Geometry: final body of the model. Coordinates: model frame, mm. Face numbers are marked on the shaded views. A direction names the side the tool comes from. Round coordinates to 2 decimals unless told otherwise and drop trailing zeros. Loops run counter-clockwise (first coordinate to the right, second up) from the corner with the lowest first, then second, coordinate; pieces in that order, holes last. Notation, with made-up numbers: (-32.75, 2) - (25.25, 2) arc R14 ccw to (25.25, 11) - close; hole circle Ø8 at (-13.5, -9). An arc over 180 degrees is marked (long way). Answer as CSV lines item,"result".
from build123d import *

# Parameters (mm, degrees)
SKETCH1_R           = 8
BOSS_EXTRUDE1_DEPTH = 3.4
SKETCH2_R           = 8
SKETCH2_R_2         = 7.6
SKETCH2_R_3         = 3.25
BOSS_EXTRUDE2_DEPTH = 1.5


with BuildPart() as part:
    # Sketch1 → Boss-Extrude1 (new body)
    with BuildSketch(Plane(origin=(0, 0, 0), x_dir=(1, 0, 0), z_dir=(0, 1, 0))):
        with Locations(Location((0, 0, 0), (0, 0, 270))):
            Circle(SKETCH1_R)
    extrude(amount=BOSS_EXTRUDE1_DEPTH)

    # Sketch2 → Boss-Extrude2 (add)
    # profile 1 of 2: a face of its own
    with BuildSketch(Plane(origin=(0, 3.4, 0), x_dir=(1, 0, 0), z_dir=(0, 1, 0))):
        with Locations(Location((0, 0, 0), (0, 0, 270))):
            Circle(SKETCH2_R)
        with Locations(Location((0, 0, 0), (0, 0, 270))):
            Circle(SKETCH2_R_2, mode=Mode.SUBTRACT)
    # profile 2 of 2: a face of its own
    with BuildSketch(Plane(origin=(0, 3.4, 0), x_dir=(1, 0, 0), z_dir=(0, 1, 0))):
        with Locations(Location((0, 0, 0), (0, 0, 270))):
            Circle(SKETCH2_R_3)
    extrude(amount=BOSS_EXTRUDE2_DEPTH)


solid = part.part
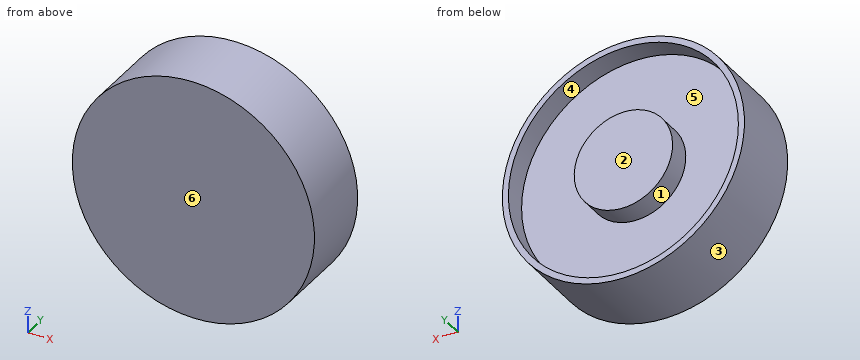
(1) Section B-B (z = 0). Output: boundary loops of the cut face in (x, y), and give its area (4 significant figures).
Findings below:
outline,"(-8, 0) - (8, 0) - (8, 4.9) - (7.6, 4.9) - (7.6, 3.4) - (3.25, 3.4) - (3.25, 4.9) - (-3.25, 4.9) - (-3.25, 3.4) - (-7.6, 3.4) - (-7.6, 4.9) - (-8, 4.9) - close"
area,"65.35 mm2"
(2) Section C-C (x = 0). Output: boundary loops of the cut face in (y, z), and give its area (4 significant figures).
Findings below:
outline,"(0, -8) - (4.9, -8) - (4.9, -7.6) - (3.4, -7.6) - (3.4, -3.25) - (4.9, -3.25) - (4.9, 3.25) - (3.4, 3.25) - (3.4, 7.6) - (4.9, 7.6) - (4.9, 8) - (0, 8) - close"
area,"65.35 mm2"
(3) Material intervals for line 1 along X through (y, z) = (3.75, 0); line 2 along Y through (x, z) = (6.25, 1); line 3 along X through (y, z) = (4.1, -1), sorted ascending.
Findings below:
line 1,"-8 to -7.6, -3.25 to 3.25, 7.6 to 8"
line 2,"0 to 3.4"
line 3,"-7.94 to -7.53, -3.09 to 3.09, 7.53 to 7.94"
(4) Section A-A (y = 4.1). Output: boundary loops of the cut face in (x, z).
Findings below:
outline,"circle Ø16 at (0, 0); circle Ø6.5 at (0, 0); hole circle Ø15.2 at (0, 0)"
(5) Access query for the marked faces 1 and 2. Directions: +Z, -Z, +X, -X, +Y, -Y. A direction counts if a zero-diameter tool reaches every point of the face in a straight line with its end or side. Return the directions, or none.
Findings below:
face 1,"+Y"
face 2,"+Z, -Z, +X, -X, +Y"
(6) Draft query along X for the marked faces 3, 4, 5 and 6. Return one class per face: pulls with the +X half, pulls with the -X half, needs draft (parallel to the pull), parting line crosses it, or undercut.
Findings below:
face 3,"parting line crosses it"
face 4,"undercut"
face 5,"undercut"
face 6,"needs draft"
(7) Pin query (flat end, axial travel): P1, Ø1, axis at y = 0.5, z = 1, coming from the +X side; P2, Ø1, axis at x = -1.5, y = 1.5, coming from the +Z side. Return the tip coordinate at first contact, or that it passes through.
Findings below:
P1,"x = 7.98"
P2,"z = 7.94"
(8) Section D-D (y = 2.15). Output: boundary loops of the cut face in (x, z), and give its area (3 significant figures).
Findings below:
outline,"circle Ø16 at (0, 0)"
area,"201 mm2"
